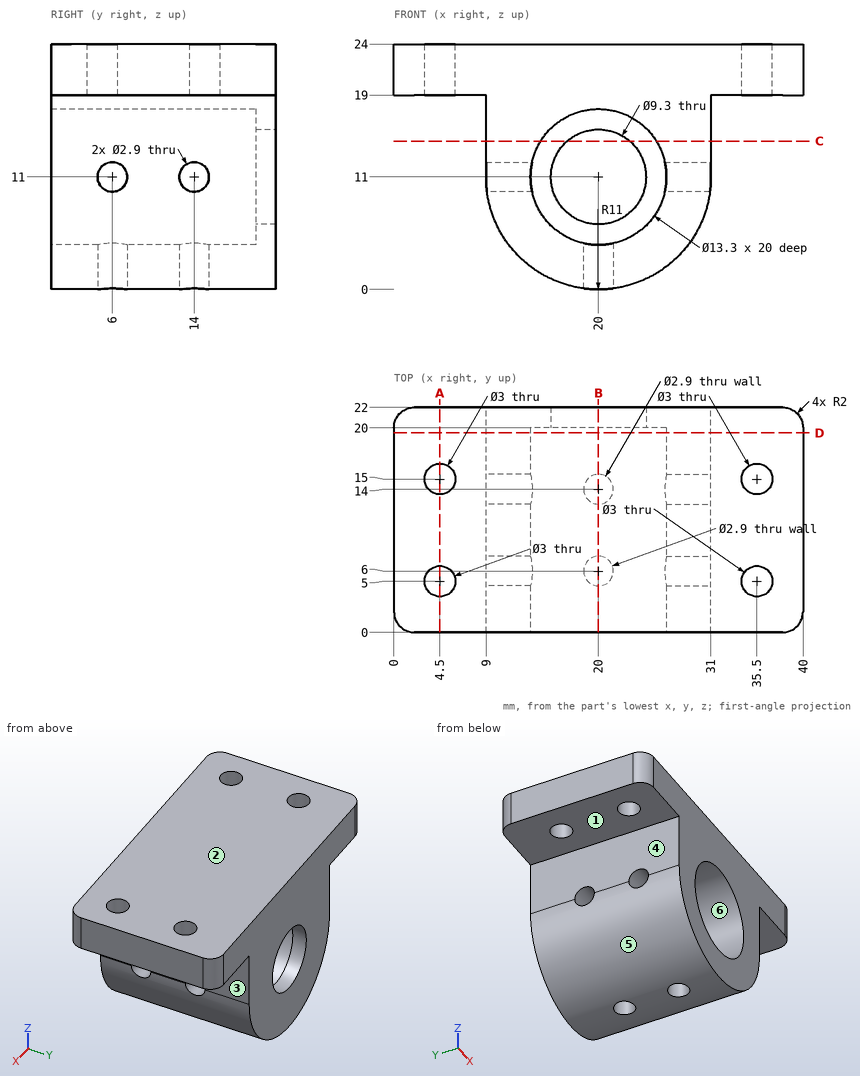
Here's the drawing with two shaded views (mm, measured from the low corner). I have some questions. A direction names the side the tool comes from. Give positions to 0.01 mm unless a question says otherwise; leave off trailing zeros. Write each loop counter-clockwise with the first axis right and the second up, starting at its lowest first coordinate (ties: lowest second). Pieces come first, ordered by that corner, then holes. Notation, with made-up numbers: (64.25, 5) - (82.25, 5) arc R15 cw to (82.25, 23) - close; hole circle Ø4 at (52, -27.75). An arc over 180 degrees is marked (long way). Write item = value, one per line. Start each with the question number.
1. Imagine slicing it at A-A (x = 4.5). Please give me the cut outline in (y, z).
2. Imagine slicing it at B-B (x = 20). Please give me the cut outline in (y, z).
3. For pin 1 (3.5 mm diameter, centred on y = 14, z = 11, fed in from -X); pin 2 (1.7 mm diameter, centred on y = 14, z = 11, fed in from +X); pin 3 (4 mm diameter, centred on y = 3, z = 5.5, fed in from -X); pin 4 (9 mm diameter, centred on y = 8, z = 13.5, fed in from +X), each with a flat end and sliding along its axis, tell me the tip position at first contact or that it passes through.
4. Please list where these lines run through material, in increasing order: line 1 (Y direction, x = 35.5, z = 20.75); line 2 (Y direction, x = 10.55, z = 11); line 3 (Z direction, x = 20, y = 16.5).
5. On a 3-axis mill with a long thin cutter (end or side, diameter ignored), from which of +Z, -Z, +X, -X, +Y, -Y can I reach the whole of each face in a straight line? I mean the marked faces 1, 2 and 3. Say none if no direction works.
6. Imagine slicing it at D-D (y = 19.5). Please give me the cut outline in (x, z), and give its area (3 significant figures).
7. Imagine slicing it at C-C (z = 14.5). Please give me the cut outline in (x, y), and give its area (3 significant figures).
8. Thinking about a two-plate mould opening in Z: for the marked faces 4, 5 and 6, which applies, released by +Z, released by -Z, zero draft, split by the parting line, or undercut?
Worked answers:
q1.outline = (0, 19) - (3.5, 19) - (3.5, 24) - (0, 24) - close; (6.5, 19) - (13.5, 19) - (13.5, 24) - (6.5, 24) - close; (16.5, 19) - (22, 19) - (22, 24) - (16.5, 24) - close
q2.outline = (0, 0) - (4.55, 0) - (4.55, 4.35) - (0, 4.35) - close; (0, 17.65) - (20, 17.65) - (20, 15.65) - (22, 15.65) - (22, 24) - (0, 24) - close; (7.45, 0) - (12.55, 0) - (12.55, 4.35) - (7.45, 4.35) - close; (15.45, 0) - (22, 0) - (22, 6.35) - (20, 6.35) - (20, 4.35) - (15.45, 4.35) - close
q3.pin_1 = 9
q3.pin_2 = through
q3.pin_3 = 9.57
q3.pin_4 = 31
q4.line_1 = 0 to 3.5, 6.5 to 13.5, 16.5 to 22
q4.line_2 = 0 to 4.55, 7.45 to 12.55, 15.45 to 22
q4.line_3 = 0 to 4.35, 17.65 to 24
q5.face_1 = -Z, -X, +Y, -Y
q5.face_2 = +Z, +X, -X, +Y, -Y
q5.face_3 = -Z, +X, +Y, -Y
q6.outline = (0, 19) - (9, 19) - (9, 11) arc R11 ccw to (31, 11) - (31, 19) - (40, 19) - (40, 24) - (0, 24) - close; hole circle Ø13.3 at (20, 11)
q6.area = 427 mm2
q7.outline = (9, 0) - (14.35, 0) - (14.35, 20) - (16.94, 20) - (16.94, 22) - (9, 22) - close; (23.06, 20) - (25.65, 20) - (25.65, 0) - (31, 0) - (31, 22) - (23.06, 22) - close
q7.area = 246 mm2
q8.face_4 = zero draft
q8.face_5 = released by -Z
q8.face_6 = undercut
